The listing builds one solid part. Answer for the finished solid, in the listing's coordinates (mm). A direction names the side the tool comes from. Give positions to 0.01 mm unless a question says otherwise; leave off trailing zeros. Write each loop counter-clockwise with the first axis right and the second up, starting at its lowest first coordinate (ties: lowest second). Pieces come first, ordered by that corner, then holes. Notation, with made-up numbers: (71, -31.75) - (77, -31.75) arc R26 cw to (77, -15.75) - close; hole circle Ø11 at (85, 22.25). An arc over 180 degrees is marked (long way). One line per question, with ' | ' between items. Start each with the question number.
1. A cutting plane is placed at B-B (y = 14.7). Determine the outline of the cut face in (x, z).
2. A cutting plane is placed at D-D (x = -13.4). Determine the outline of the cut face in (y, z).
3. For faces 5 (the face through (-15, 15, -10)), 6 (the face through (-14.446, 13.935, -4.93)), 7 (the face through (-14.04, 14.43, 2.01)), determine the directions among +Z, -Z, +X, -X, +Y, -Y from which every point of the face is accessible in a straight line to the end or side of a thin tool.
4. A cutting plane is placed at A-A (x = -15). Determine the outline of the cut face in (y, z).
5. A cutting plane is placed at C-C (z = -2). Determine the outline of the cut face in (x, y), then the cut area to 3 significant figures.
6. Given P1, Ø1, axis at y = 16, z = 1.5, coming from the -X side; P2, Ø2, axis at x = -14, z = 1.5, coming from the -Y side; P3, Ø2, axis at x = -16, z = -4, coming from the +Y side; P4, Ø1.1, axis at x = -15, y = 15, coming from the +Z side, each flat-ended and moving along its own axis, determine where each tip first touches the part or whether it passes through.
7. Find the intervals of material crossed by L1, parallel to Z at x = -15.1, y = 14.3; L2, parallel to Z at x = -13.4, y = 15.8; L3, parallel to X at y = 14.15, z = -3.25, in increasing order. Write a range as from..to.
8. The mould has two halves that part along Y. Classify faces 1 (the face through (-15.96, 15.57, 2.01)), 2 (the face through (-14.028, 15.551, 2.014)), 3 (the face through (-15, 17, 1)), 4 (the face through (-14, 14, 0)): +Y half, -Y half, draft (parallel to the pull), parting line (faces both ways), or undercut.
```python
from build123d import *

# Parameters (mm, degrees)
SKETCH1_R           = 1.2
BOSS_EXTRUDE1_DEPTH = 10
SKETCH2_R           = 2
BOSS_EXTRUDE2_DEPTH = 3
CUT_EXTRUDE1_DEPTH  = 2


with BuildPart() as part:
    # Sketch1 → Boss-Extrude1 (new body)
    with BuildSketch(Plane.XY):
        with Locations((-15, 15)):
            Circle(SKETCH1_R)
    extrude(amount=-BOSS_EXTRUDE1_DEPTH)

    # Sketch2 → Boss-Extrude2 (add)
    with BuildSketch(Plane.XY):
        with Locations((-15, 15)):
            Circle(SKETCH2_R)
    extrude(amount=BOSS_EXTRUDE2_DEPTH)

    # Sketch3 → Cut-Extrude1 (cut)
    with BuildSketch(Plane.XY.offset(3)):
        Polygon((-13.709947687, 15), (-14.354973843, 16.117218076), (-15.645026157, 16.117218076), (-16.290052313, 15), (-15.645026157, 13.882781924), (-14.354973843, 13.882781924), align=None)
    extrude(amount=-CUT_EXTRUDE1_DEPTH, mode=Mode.SUBTRACT)


solid = part.part
```
Determined:
1) outline: (-16.98, 0) - (-16.16, 0) - (-16.16, -10) - (-13.84, -10) - (-13.84, 0) - (-13.02, 0) - (-13.02, 3) - (-13.88, 3) - (-13.88, 1) - (-16.12, 1) - (-16.12, 3) - (-16.98, 3) - close
2) outline: (13.8, 0) - (16.2, 0) - (16.2, 3) - (13.8, 3) - close
3) face 5: -Z, +X, -X, +Y, -Y | face 6: -Z | face 7: +Z
4) outline: (13, 0) - (13.8, 0) - (13.8, -10) - (16.2, -10) - (16.2, 0) - (17, 0) - (17, 3) - (16.12, 3) - (16.12, 1) - (13.88, 1) - (13.88, 3) - (13, 3) - close
5) outline: circle Ø2.4 at (-15, 15) | area: 4.52 mm2
6) P1: x = -16.94 | P2: y = 13 | P3: y = 16.2 | P4: z = 1
7) L1: -10..1 | L2: 0..3 | L3: -15.85..-14.15
8) face 1: undercut | face 2: undercut | face 3: parting line | face 4: draft
